from build123d import *

# Parameters (mm, degrees)
F0_R     = 2.65
F0_W     = 78.782992
F0_H     = 20
F1_DEPTH = 3


with BuildPart() as f1:
    # F0 (on Right) → F1 (new body)
    with BuildSketch(Plane.YZ):
        Polygon((280, -270), (280, -260), (280, 214), (201.217008, 214), (201.217008, 280), (201.217008, 300), (-201.217008, 300), (-201.217008, 280), (-201.217008, 214), (-280, 214), (-280, -270), (-43, -270), (-43, -238), (-24, -238), (-24, -212), (24, -212), (24, -238), (43, -238), (43, -270), align=None)
        with Locations((-260, -250)):
            Circle(F0_R, mode=Mode.SUBTRACT)
        with Locations((260, -250)):
            Circle(F0_R, mode=Mode.SUBTRACT)
        with Locations((240.608504, 290)):
            Rectangle(F0_W, F0_H)
        with Locations((-240.608504, 290)):
            Rectangle(F0_W, F0_H)
    extrude(amount=F1_DEPTH)


solid = f1.part
Here's how the part is built. I have some questions about the finished solid (model axes, mm). Round coordinates to 2 decimals unless told otherwise and drop trailing zeros. Order: outer loops, then holes, each group sorted by start corner. A loop starts at its lowest first (then second) coordinate and runs counter-clockwise, first axis right, second up. Notation, with made-up numbers: M 71,60 L 89,60 A28 ccw 89,97 Z; hole C -5,-14.5 d10. An arc over 180 degrees is marked long. Return JSON: item names as keys, results as strings. Group by question number.
1. Please list where these lines run through material, in increasing order: probe 1 along Y at (x, z) = (1.75, -250); probe 2 along Z at (x, y) = (1.35, -260); probe 3 along Z at (x, y) = (0.7, -243).
2. If we mould it in two halves opening along X, with no side actions, what happens to faces 1 (the face through (0, -4, 19)), 2 (the face through (3, -4, 19))? For each: pulls with the +X half, pulls with the -X half, needs draft (parallel to the pull), parting line crosses it, or undercut.
3. If we section it at C-C on y = 17: List the corners of the cut face in (x, z) for me, then the cut area to 3 significant figures.
4. I'm going to push flat-ended pins straight in: pin 1 Ø6 at (y, z) = (-260, -250) entering from -X; pin 2 Ø1.5 at (x, y) = (2, 31.5) entering from -Z; pin 3 Ø1.5 at (x, y) = (1.5, 6.5) entering from -Z. Where does each tip first touch, or does it pass through?
5. If we section it at A-A on x = 0.95: List the corners of the cut face in (y, z) for me.
6. If we section it at B-B on y = -236: List the corners of the cut face in (x, z) for me, then the cut area to 3 significant figures.
Reply:
{
 "1": {"probe 1": "-280 to -262.65, -257.35 to -43, 43 to 257.35, 262.65 to 280", "probe 2": "-270 to -252.65, -247.35 to 214, 280 to 300", "probe 3": "-270 to 214, 280 to 300"},
 "2": {"face 1": "pulls with the -X half", "face 2": "pulls with the +X half"},
 "3": {"outline": "M 0,-212 L 3,-212 L 3,300 L 0,300 Z", "area": "1,540 mm^2"},
 "4": {"pin 1": "x = 0", "pin 2": "z = -238", "pin 3": "z = -212"},
 "5": {"outline": "M -280,-270 L -43,-270 L -43,-238 L -24,-238 L -24,-212 L 24,-212 L 24,-238 L 43,-238 L 43,-270 L 280,-270 L 280,214 L 201.22,214 L 201.22,280 L 280,280 L 280,300 L -280,300 L -280,280 L -201.22,280 L -201.22,214 L -280,214 Z; hole C -260,-250 d5.3; hole C 260,-250 d5.3"},
 "6": {"outline": "M 0,-270 L 3,-270 L 3,214 L 0,214 Z; M 0,280 L 3,280 L 3,300 L 0,300 Z", "area": "1,510 mm^2"}
}
